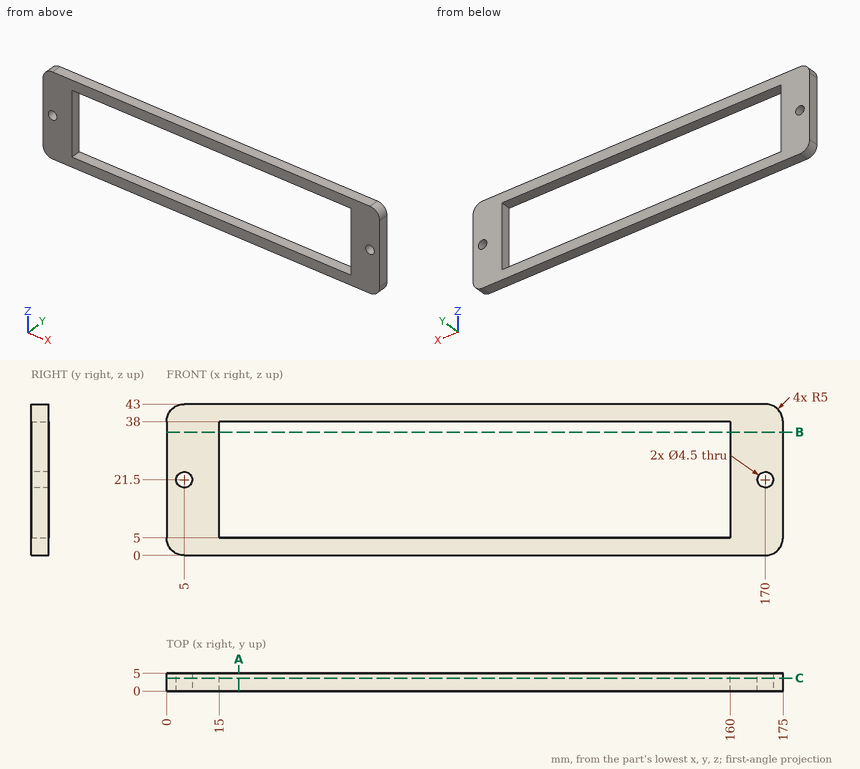
For this review, use the dimensioned drawing (mm, ordinates from the lowest corner) and the shaded views. Give positions to 0.01 mm unless a question says otherwise; leave off trailing zeros. Order: outer loops, then holes, each group sorted by start corner. A loop starts at its lowest first (then second) coordinate and runs counter-clockwise, first axis right, second up. Notation, with made-up numbers: (62.5, 12) - (120.5, 12) arc R13 ccw to (120.5, 16) - close; hole circle Ø8 at (9.25, 43.25). An arc over 180 degrees is marked (long way). Use a Markdown table: item, result. Add a question column.
(1) Add section C-C on y = 3.7. Give the boundary of the cut face in (x, z).
(2) Add section A-A on x = 20.5. Give the boundary of the cut face in (y, z).
(3) Wall thickness on probe 1 along Z at (x, y) = (156.5, 3.3); probe 2 along X at (y, z) = (4.55, 10.5); probe 3 along X at (y, z) = (1.75, 20.5): over which ranges is each line inside the solid? List them lowest first. Write a range as [from, to].
(4) Add section B-B on z = 35. Give the boundary of the cut face in (x, y), then the cut area to 3 significant figures.
Report:
| question | item | result |
|---|---|---|
| 1 | outline | (0, 5) arc R5 ccw to (5, 0) - (170, 0) arc R5 ccw to (175, 5) - (175, 38) arc R5 ccw to (170, 43) - (5, 43) arc R5 ccw to (0, 38) - close; hole circle Ø4.5 at (5, 21.5); hole (15, 5) - (160, 5) - (160, 38) - (15, 38) - close; hole circle Ø4.5 at (170, 21.5) |
| 2 | outline | (0, 0) - (5, 0) - (5, 5) - (0, 5) - close; (0, 38) - (5, 38) - (5, 43) - (0, 43) - close |
| 3 | probe 1 | z = [0, 5], [38, 43] |
| 3 | probe 2 | x = [0, 15], [160, 175] |
| 3 | probe 3 | x = [0, 2.98], [7.02, 15], [160, 167.98], [172.02, 175] |
| 4 | outline | (0, 0) - (15, 0) - (15, 5) - (0, 5) - close; (160, 0) - (175, 0) - (175, 5) - (160, 5) - close |
| 4 | area | 150 mm² |
